Part model, mm, in its own coordinate system. Face numbers are marked on the shaded views. Give positions to 0.01 mm unless a question says otherwise; leave off trailing zeros. Order: outer loops, then holes, each group sorted by start corner. A loop starts at its lowest first (then second) coordinate and runs counter-clockwise, first axis right, second up. Notation, with made-up numbers: (29.25, 53.5) - (35.25, 53.5) arc R26 cw to (35.25, 89.5) - close; hole circle Ø3 at (22.25, -27). An arc over 180 degrees is marked (long way). Use a Markdown table: item, result. Add a question column.
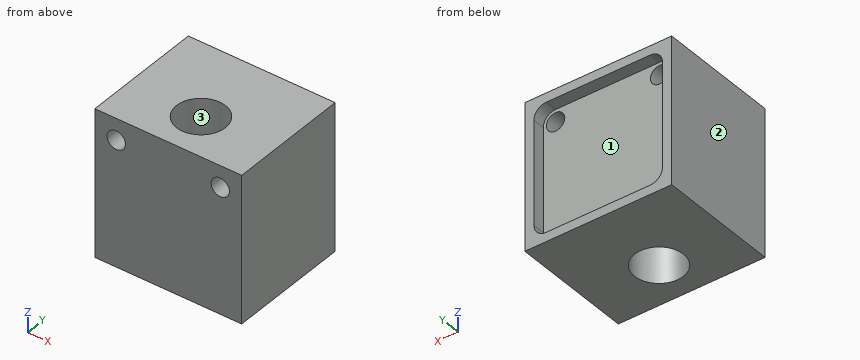
from build123d import *

# Parameters (mm, degrees)
SKETCH1_W           = 24
SKETCH1_H           = 24
BOSS_EXTRUDE1_DEPTH = 20
SKETCH2_W           = 21
SKETCH2_H           = 21
CUT_EXTRUDE1_DEPTH  = 2
FILLET2_R           = 2
SKETCH3_R           = 4
CUT_EXTRUDE2_DEPTH  = 42
SKETCH5_R           = 1.5
CUT_EXTRUDE3_DEPTH  = 42


with BuildPart() as part:
    # Sketch1 → Boss-Extrude1 (new body)
    with BuildSketch(Plane(origin=(0, 0, 0), x_dir=(1, 0, 0), z_dir=(0, 1, 0))):
        Rectangle(SKETCH1_W, SKETCH1_H)
    extrude(amount=BOSS_EXTRUDE1_DEPTH)

    # Sketch2 → Cut-Extrude1 (cut)
    with BuildSketch(Plane(origin=(0, 20, 0), x_dir=(1, 0, 0), z_dir=(0, 1, 0))):
        Rectangle(SKETCH2_W, SKETCH2_H)
    extrude(amount=-CUT_EXTRUDE1_DEPTH, mode=Mode.SUBTRACT)

    # Fillet2
    fillet2_edges = [part.edges().sort_by_distance(p)[0] for p in [
        (10.5, 19, -10.5),
        (10.5, 19, 10.5),
        (-10.5, 19, 10.5),
        (-10.5, 19, -10.5),
    ]]
    fillet(fillet2_edges, radius=FILLET2_R)

    # Sketch3 → Cut-Extrude2 (cut)
    with BuildSketch(Plane.XY.offset(12)):
        with Locations((0, 7)):
            Circle(SKETCH3_R)
    extrude(amount=-CUT_EXTRUDE2_DEPTH, mode=Mode.SUBTRACT)

    # Sketch5 → Cut-Extrude3 (cut)
    with BuildSketch(Plane(origin=(0, 18, 0), x_dir=(1, 0, 0), z_dir=(0, 1, 0))):
        with Locations(Location((-8.5, -8.5, 0), (0, 0, 270))):
            Circle(SKETCH5_R)
        with Locations(Location((8.5, -8.5, 0), (0, 0, 270))):
            Circle(SKETCH5_R)
    extrude(amount=-CUT_EXTRUDE3_DEPTH, mode=Mode.SUBTRACT)


solid = part.part
1. Cut at B-B (y = 9.75). Write the cut outline in (x, z), plus the area to 3 significant figures.
2. Pin check, flat tip, straight feed: P1, Ø10, axis at x = -1, z = 1, coming from the +Y side. Stop position of the tip, or through.
3. Cut at D-D (x = 4.75). Write the cut outline in (y, z), plus the area to 3 significant figures.
4. Cut at A-A (x = 0). Write the cut outline in (y, z).
5. Mould opens along Y. For the marked faces 1, 2 and 3 say: released by +Y, released by -Y, zero draft, split by the parting line, or undercut.
6. Drill centre lines: probe 1 along X at (y, z) = (13, 8.5); probe 2 along X at (y, z) = (6.25, 8.5); probe 3 along Y at (x, z) = (0, -0.75). Where is each one in solid material? Low to high. Write a range as [from, to].
7. Cut at C-C (z = 5). Write the cut outline in (x, y).
Responses:
| question | item | result |
|---|---|---|
| 1 | outline | (-12, -12) - (-2.9, -12) - (-2.9, 12) - (-12, 12) - close; (2.9, -12) - (12, -12) - (12, 12) - (2.9, 12) - close; hole circle Ø3 at (-8.5, 8.5); hole circle Ø3 at (8.5, 8.5) |
| 1 | area | 422 mm² |
| 2 | P1 | stops at y = 18 |
| 3 | outline | (0, -12) - (20, -12) - (20, -10.5) - (18, -10.5) - (18, 10.5) - (20, 10.5) - (20, 12) - (0, 12) - close |
| 3 | area | 438 mm² |
| 4 | outline | (0, -12) - (3, -12) - (3, 12) - (0, 12) - close; (11, -12) - (20, -12) - (20, -10.5) - (18, -10.5) - (18, 10.5) - (20, 10.5) - (20, 12) - (11, 12) - close |
| 5 | face 1 | released by +Y |
| 5 | face 2 | zero draft |
| 5 | face 3 | undercut |
| 6 | probe 1 | x = [-12, -10], [-7, 7], [10, 12] |
| 6 | probe 2 | x = [-12, -10], [-7, -3.93], [3.93, 7], [10, 12] |
| 6 | probe 3 | y = [0, 3], [11, 18] |
| 7 | outline | (-12, 0) - (12, 0) - (12, 20) - (10.5, 20) - (10.5, 18) - (-10.5, 18) - (-10.5, 20) - (-12, 20) - close; hole circle Ø8 at (0, 7) |
